from build123d import *

# Parameters (mm, degrees)
SKETCH1_R                                      = 0.5
SKETCH1_R_2                                    = 5.25
BOSS_EXTRUDE1_DEPTH                            = 5
SKETCH3_R                                      = 1.3
BOSS_EXTRUDE4_DEPTH                            = 5.7
BOSS_EXTRUDE6_DEPTH                            = 2.473491095
FILLET1_R                                      = 2.5
FILLET2_R                                      = 2
F_2_0MM_DOWEL_HOLE1_D                          = 2
F_2_0MM_DOWEL_HOLE1_DEPTH                      = 42.93
F_2_0MM_DOWEL_HOLE1_TIP                        = 0.600860619
CSK_FOR_M2_5_FLAT_HEAD_MACHINE_SCREW1_AT_COUNT = 2
CSK_FOR_M2_5_FLAT_HEAD_MACHINE_SCREW1_AT_PITCH = 28
SKETCH14_R                                     = 2.75
CUT_EXTRUDE1_DEPTH                             = 27.54536008


with BuildPart() as part:
    # Sketch1 → Boss-Extrude1 (new body)
    with BuildSketch(Plane(origin=(0, 0, 0), x_dir=(1, 0, 0), z_dir=(0, 1, 0))):
        with BuildLine():
            Line((1.767766953, 15.096194078), (15.096194078, 1.767766953))
            ThreePointArc((15.096194078, 1.767766953), (15.828427125, 0), (15.096194078, -1.767766953))
            Line((15.096194078, -1.767766953), (1.767766953, -15.096194078))
            ThreePointArc((1.767766953, -15.096194078), (0, -15.828427125), (-1.767766953, -15.096194078))
            Line((-1.767766953, -15.096194078), (-15.096194078, -1.767766953))
            ThreePointArc((-15.096194078, -1.767766953), (-15.828427125, 0), (-15.096194078, 1.767766953))
            Line((-15.096194078, 1.767766953), (-1.767766953, 15.096194078))
            ThreePointArc((-1.767766953, 15.096194078), (0, 15.828427125), (1.767766953, 15.096194078))
        make_face()
        with Locations(Location((0, 10.5, 0), (0, 0, 270))):
            Circle(SKETCH1_R, mode=Mode.SUBTRACT)
        with Locations(Location((0, -10.5, 0), (0, 0, 270))):
            Circle(SKETCH1_R, mode=Mode.SUBTRACT)
        with Locations(Location((10.5, 0, 0), (0, 0, 270))):
            Circle(SKETCH1_R, mode=Mode.SUBTRACT)
        with Locations(Location((-10.5, 0, 0), (0, 0, 270))):
            Circle(SKETCH1_R, mode=Mode.SUBTRACT)
        with Locations(Location((0, 0, 0), (0, 0, 270))):
            Circle(SKETCH1_R_2, mode=Mode.SUBTRACT)
    extrude(amount=BOSS_EXTRUDE1_DEPTH)

    # Sketch3 → Boss-Extrude4 (add)
    # profile 1 of 4: a face of its own
    with BuildSketch(Plane(origin=(0, -2.7, 0), x_dir=(1, 0, 0), z_dir=(0, 1, 0))):
        Polygon((-4.949747468, -10.537489101), (-0.637994164, -14.849242405), (-4.949747468, -19.160995709), (-9.261500772, -14.849242405), align=None)
        with Locations(Location((-4.949747468, -14.849242405, 0), (0, 0, 90))):
            Circle(SKETCH3_R, mode=Mode.SUBTRACT)
    # profile 2 of 4: a face of its own
    with BuildSketch(Plane(origin=(0, -2.7, 0), x_dir=(1, 0, 0), z_dir=(0, 1, 0))):
        Polygon((-6.717514421, -8.769722148), (-11.029267725, -13.081475452), (-9.261500772, -14.849242405), (-4.949747468, -10.537489101), align=None)
    # profile 3 of 4: a face of its own
    with BuildSketch(Plane(origin=(0, -2.7, 0), x_dir=(1, 0, 0), z_dir=(0, 1, 0))):
        Polygon((19.160995709, 4.949747468), (14.849242405, 9.261500772), (10.537489101, 4.949747468), (14.849242405, 0.637994164), align=None)
        with Locations(Location((14.849242405, 4.949747468, 0), (0, 0, 90))):
            Circle(SKETCH3_R, mode=Mode.SUBTRACT)
    # profile 4 of 4: a face of its own
    with BuildSketch(Plane(origin=(0, -2.7, 0), x_dir=(1, 0, 0), z_dir=(0, 1, 0))):
        Polygon((13.081475452, 11.029267725), (14.849242405, 9.261500772), (10.537489101, 4.949747468), (8.769722148, 6.717514421), align=None)
    extrude(amount=BOSS_EXTRUDE4_DEPTH)


with BuildPart() as boss_extrude6_tool:
    # Sketch7 → Boss-Extrude6 (new body)
    with BuildSketch(Plane(origin=(2.775126076, -2.11e-07, 2.775126076), x_dir=(0.7071067811865474, 0, -0.7071067811865478), z_dir=(0.7071067811865468, -5.372690076738491e-08, 0.7071067811865464))):
        Polygon((11.924621202, 5.000000506), (17.04887, 3.00000054), (11.924621202, 3.000000506), align=None)
        Polygon((-11.924621202, 5.000000506), (-17.04887, 3.00000054), (-11.924621202, 3.000000506), align=None)
    extrude(amount=-BOSS_EXTRUDE6_DEPTH)


with BuildPart() as part_1:
    add(part.part)


with BuildPart() as part_2:
    # Boss-Extrude6: joined with boss_extrude6_tool
    add(part_1.part.fuse(boss_extrude6_tool.part, tol=0.00001))

    # Fillet1
    fillet1_edges = [part_2.edges().sort_by_distance(p)[0] for p in [
        (-7.405876652, 1.5, 9.458084379),
        (-1.270359497, 1.5, 15.481607737),
        (9.458084379, 1.5, -7.405876652),
        (15.481607737, 1.5, -1.270359497),
    ]]
    fillet(fillet1_edges, radius=FILLET1_R)

    # Fillet2
    # the kernel refuses this fillet: 2 mm, written as the material it takes off along each edge
    with BuildSketch(Plane(origin=(-4.949747468, -7.7, 19.160995709), x_dir=(0.7071067811865477, 0, -0.7071067811865475), z_dir=(0, 1, 0)), Plane(origin=(13.081475452, -7.7, -11.029267725), x_dir=(-0.7071067811865471, 0, 0.707106781186548), z_dir=(0, 1, 0)), Plane(origin=(19.160995709, -7.7, -4.949747468), x_dir=(-0.7071067811865482, 0, -0.7071067811865469), z_dir=(0, 1, 0))) as fillet2_piece_1:
        with BuildLine():
            CenterArc((FILLET2_R, FILLET2_R), FILLET2_R, 180, 90)
            Line((0, FILLET2_R), (0, 0))
            Line((0, 0), (FILLET2_R, 0))
        make_face()
    extrude(amount=15.7, mode=Mode.SUBTRACT)
    with BuildSketch(Plane(origin=(-11.029267725, -7.7, 13.081475452), x_dir=(0.7071067811865476, 0, -0.7071067811865476), z_dir=(0, 1, 0))) as fillet2_piece_2:
        with BuildLine():
            CenterArc((FILLET2_R, -FILLET2_R), FILLET2_R, 90, 90)
            Line((0, -FILLET2_R), (0, 0))
            Line((0, 0), (FILLET2_R, 0))
        make_face()
    extrude(amount=15.7, mode=Mode.SUBTRACT)

    # Ø2.0mm Dowel Hole1
    with Locations(Plane.XZ):
        with Locations((0, 10.5), (10.5, 0), (-10.5, 0), (0, -10.5)):
            Hole(F_2_0MM_DOWEL_HOLE1_D / 2, depth=F_2_0MM_DOWEL_HOLE1_DEPTH)
            with Locations((0, 0, -(F_2_0MM_DOWEL_HOLE1_DEPTH + F_2_0MM_DOWEL_HOLE1_TIP / 2))):  # 118° drill point
                Cone(0, F_2_0MM_DOWEL_HOLE1_D / 2, F_2_0MM_DOWEL_HOLE1_TIP, mode=Mode.SUBTRACT)

    # Sketch12 → CSK for M2.5 Flat Head Machine Screw1 (revolve, cut)
    with BuildSketch(Plane(origin=(-4.949747468, 3, 14.849242405), x_dir=(0, 0, 1), z_dir=(1, 0, 0))):
        Polygon((0, 0), (0, 5.7), (1.35, 5.7), (1.35, 1.4), (2.75, 0), align=None)
    csk_for_m2_5_flat_head_machine_screw1 = revolve(axis=Axis((-4.949747468, 9.35, 14.849242405), (0, -1, 0)), mode=Mode.SUBTRACT)

    # CSK for M2.5 Flat Head Machine Screw1 at: CSK for M2.5 Flat Head Machine Screw1 ×2
    with Locations(*[Vector(0.7071067811865477, 0, -0.7071067811865475) * (i * CSK_FOR_M2_5_FLAT_HEAD_MACHINE_SCREW1_AT_PITCH) for i in range(1, CSK_FOR_M2_5_FLAT_HEAD_MACHINE_SCREW1_AT_COUNT)]):
        add(csk_for_m2_5_flat_head_machine_screw1, mode=Mode.SUBTRACT)

    # Sketch14 → Cut-Extrude1 (cut, through all)
    with BuildSketch(Plane(origin=(0, 3, 0), x_dir=(1, 0, 0), z_dir=(0, 1, 0))):
        with Locations((-4.949747468, -14.849242405)):
            Circle(SKETCH14_R)
        with Locations((14.849242405, 4.949747468)):
            Circle(SKETCH14_R)
    extrude(amount=CUT_EXTRUDE1_DEPTH, mode=Mode.SUBTRACT)


solid = part_2.part
The listing builds one solid part. Answer for the finished solid, in the listing's coordinates (mm). A direction names the side the tool comes from. Round coordinates to 2 decimals unless told otherwise and drop trailing zeros. Order: outer loops, then holes, each group sorted by start corner. A loop starts at its lowest first (then second) coordinate and runs counter-clockwise, first axis right, second up. Notation, with made-up numbers: (55, 81.25) -> (68, 81.25) arc R33 ccw to (68, 115.25) -> close; hole circle Ø5 at (85, 74.25). An arc over 180 degrees is marked (long way). One line per item, written item: value.
Item 1: Find section C-C, the plane y = 2.5. State how many separate pieces and enclosed holes the cut face has, then the cut area to 3 significant figures.
Taken from the geometry:
separate pieces: 1
enclosed holes: 7
area: 520 mm2
Item 2: For faces 4 (the flat face through (16.6, -0.52, -2.39)), 5 (the flat face through (-6.69, 3.57, 12.24)), 6 (the flat face through (-12.093, 2.465, 4.771)), 7 (the cylindrical face through (13.1, 0.5, -10.2)), determine the directions among +Z, -Z, +X, -X, +Y, -Y from which every point of the face is accessible in a straight line to the end or side of a thin tool.
Taken from the geometry:
face 4: +Z, +X, -Y
face 5: +Z, +Y
face 6: -X, +Y, -Y
face 7: -Z, +Y, -Y
Item 3: For a pull along Z with two mould halves and no side action, classify faces 1 (the cylindrical face through (-15.83, 2.46, 0.03)), 2 (the flat face through (-7.97, 0.11, 16.14)), 3 (the flat face through (12.24, 3.57, -6.69)) as released by +Z, released by -Z, zero draft, split by the parting line, or undercut.
Taken from the geometry:
face 1: split by the parting line
face 2: released by +Z
face 3: undercut
Item 4: Find section B-B, the plane y = -1.75. Give the vertices of the cut face in (x, z).
Taken from the geometry:
outline: (-9.62, 11.67) -> (-6.72, 8.77) -> (-0.64, 14.85) -> (-3.54, 17.75) arc R2 ccw to (-6.36, 17.75) -> (-9.62, 14.5) arc R2 ccw to start; (8.77, -6.72) -> (11.67, -9.62) arc R2 ccw to (14.5, -9.62) -> (17.75, -6.36) arc R2 ccw to (17.75, -3.54) -> (14.85, -0.64) -> close; hole circle Ø2.7 at (-4.95, 14.85); hole circle Ø2.7 at (14.85, -4.95)
Item 5: Find section D-D, the plane x = 10.5. Give the vertices of the cut face in (y, z), then the cut area to 3 significant figures.
Taken from the geometry:
outline: (-2.7, -8.45) -> (0, -8.45) -> (0, -8.67) -> (4.36, -8.67) -> (5, -6.36) -> (5, -1) -> (0, -1) -> (0, -4.99) -> (-2.7, -4.99) -> close; (0, 1) -> (5, 1) -> (5, 6.36) -> (0, 6.36) -> close
area: 73.8 mm2
Item 6: Find section A-A, the plane z = 10.5. Give the vertices of the cut face in (x, y).
Taken from the geometry:
outline: (-8.67, 0) -> (-8.45, 0) -> (-8.45, -2.7) -> (-4.99, -2.7) -> (-4.99, 0) -> (-1, 0) -> (-1, 5) -> (-6.36, 5) -> (-8.67, 4.36) -> close; (1, 0) -> (6.36, 0) -> (6.36, 5) -> (1, 5) -> close
Item 7: Given P1, Ø4, axis at x = 2, z = 8, coming from the -Y side; P2, Ø3, axis at x = -4.95, z = 14.85, coming from the +Y side; P3, Ø4.5, axis at x = 14.85, z = -4.95, coming from the +Y side; P4, Ø1.6, axis at x = 0, z = 10.5, coming from the +Y side, each flat-ended and moving along its own axis, determine where each tip first touches the part or whether it passes through.
Taken from the geometry:
P1: stops at y = 0
P2: stops at y = 1.75
P3: stops at y = 2.5
P4: passes through
Item 8: Straight lines are drawn through the part: L1, parallel to Y at x = -8, z = -1.5; L2, parallel to X at y = 4, z = -4; L3, parallel to Z at x = 3, y = 1.5. For each, find the intervals that lie inside material, in ascending order.
Taken from the geometry:
L1: y = 0 to 5
L2: x = -12.86 to -3.4, 3.4 to 12.27
L3: z = -13.86 to -4.31, 4.31 to 13.86
